```python
from build123d import *

# Parameters (mm, degrees)
SKETCH1_R                       = 32.5
EXTRUDE1_DEPTH                  = 18.9992
CHAMFER1_SIZE                   = 4.57
M3X0_5_TAPPED_HOLE3_D           = 2.5
M3X0_5_TAPPED_HOLE3_DEPTH       = 7.8486
M3X0_5_TAPPED_HOLE3_CBORE_D     = 3
M3X0_5_TAPPED_HOLE3_CBORE_DEPTH = 6.35
M3X0_5_TAPPED_HOLE3_TIP         = 0.751075774
M5X0_8_TAPPED_HOLE1_D           = 4.2
M5X0_8_TAPPED_HOLE1_DEPTH       = 27.94
M5X0_8_TAPPED_HOLE1_CBORE_D     = 5
M5X0_8_TAPPED_HOLE1_CBORE_DEPTH = 7.62
M5X0_8_TAPPED_HOLE1_TIP         = 1.2618073
HOLE1_D                         = 3.048
HOLE1_DEPTH                     = 6.35
HOLE1_CBORE_D                   = 7.874
HOLE1_CBORE_DEPTH               = 0.254
HOLE1_TIP                       = 0.915711583
SKETCH2_R                       = 31.6865
EXTRUDE2_DEPTH                  = 1.00076


with BuildPart() as part:
    # Sketch1 → Extrude1 (new body)
    with BuildSketch(Plane(origin=(0, 0, 0), x_dir=(1, 0, 0), z_dir=(0, 1, 0))):
        with Locations(Location((0, 0, 0), (0, 0, 270))):  # turned: the seam where the file's is
            Circle(SKETCH1_R)
    extrude(amount=EXTRUDE1_DEPTH)

    # Sketch3 → Cut-Revolve1 (revolve, cut)
    with BuildSketch(Plane.XY, mode=Mode.PRIVATE) as cut_revolve1_sk:
        with BuildLine():
            Line((2.3876, 13.463763428), (2.3876, 12.7508))
            Line((2.3876, 12.7508), (0, 12.7508))
            Line((0, 12.7508), (0, 18.9992))
            Line((0, 18.9992), (6.470525878, 18.9992))
            ThreePointArc((6.470525878, 18.9992), (5.220905936, 15.647420055), (2.3876, 13.463763428))
        make_face()
    revolve(cut_revolve1_sk.sketch.rotate(Axis((0, 18.9992, 0), (0, -1, 0)), 90), axis=Axis((0, 18.9992, 0), (0, -1, 0)), mode=Mode.SUBTRACT)  # turned: the seam where the file's is

    # Chamfer1
    chamfer1_edges = [part.edges().sort_by_distance(p)[0] for p in [
        (0, 18.9992, -32.5),
    ]]
    chamfer(chamfer1_edges, length=CHAMFER1_SIZE)

    # M3x0.5 Tapped Hole3
    with Locations(Plane(origin=(0, 18.9992, 0), x_dir=(-1, 0, 0), z_dir=(0, 1, 0))):
        with Locations((-5.3975, -9.348744234), (10.795, 0), (-5.3975, 9.348744234)):
            CounterBoreHole(M3X0_5_TAPPED_HOLE3_D / 2, M3X0_5_TAPPED_HOLE3_CBORE_D / 2, M3X0_5_TAPPED_HOLE3_CBORE_DEPTH, depth=M3X0_5_TAPPED_HOLE3_DEPTH)
            with Locations((0, 0, -(M3X0_5_TAPPED_HOLE3_DEPTH + M3X0_5_TAPPED_HOLE3_TIP / 2))):  # 118° drill point
                Cone(0, M3X0_5_TAPPED_HOLE3_D / 2, M3X0_5_TAPPED_HOLE3_TIP, mode=Mode.SUBTRACT)

    # M5x0.8 Tapped Hole1
    with Locations(Plane(origin=(32.5, 6.6802, 0), x_dir=(0, 0, 1), z_dir=(1, 0, 0))):
        with Locations((0, 0)):
            CounterBoreHole(M5X0_8_TAPPED_HOLE1_D / 2, M5X0_8_TAPPED_HOLE1_CBORE_D / 2, M5X0_8_TAPPED_HOLE1_CBORE_DEPTH, depth=M5X0_8_TAPPED_HOLE1_DEPTH)
            with Locations((0, 0, -(M5X0_8_TAPPED_HOLE1_DEPTH + M5X0_8_TAPPED_HOLE1_TIP / 2))):  # 118° drill point
                Cone(0, M5X0_8_TAPPED_HOLE1_D / 2, M5X0_8_TAPPED_HOLE1_TIP, mode=Mode.SUBTRACT)

    # Hole1
    with Locations(Plane(origin=(32.5, 6.6802, 0), x_dir=(0, 0, 1), z_dir=(1, 0, 0))):
        with Locations((0, 0)):
            CounterBoreHole(HOLE1_D / 2, HOLE1_CBORE_D / 2, HOLE1_CBORE_DEPTH, depth=HOLE1_DEPTH)
            with Locations((0, 0, -(HOLE1_DEPTH + HOLE1_TIP / 2))):  # 118° drill point
                Cone(0, HOLE1_D / 2, HOLE1_TIP, mode=Mode.SUBTRACT)

    # Sketch2 → Extrude2 (add)
    with BuildSketch(Plane.XZ):
        with Locations(Location((0, 0, 0), (0, 0, 90))):  # turned: the seam where the file's is
            Circle(SKETCH2_R)
    extrude(amount=EXTRUDE2_DEPTH)


solid = part.part
```
Geometry check sheet. Reference: the model listing, model coordinates, mm. A direction names the side the tool comes from. Coordinates: 2 decimals unless noted, no trailing zeros. Put each result on its own line as item: value.
1) Thickness scan on line 1 (Y direction, x = 27.25, z = 0); line 2 (Y direction, x = 32.3, z = 0); line 3 (Z direction, x = 29.5, y = 5.25). Record the ranges inside material, lowest first.
Result set:
line 1: y = -1 to 4.18, 9.18 to 19
line 2: y = 0 to 2.74, 10.62 to 14.63
line 3: z = -13.64 to -2.05, 2.05 to 13.64
2) Gauge pin test, flat ends, axial feed: pin 1 Ø4 at (x, y) = (8.5, 5.5) entering from +Z; pin 2 Ø5.5 at (y, z) = (6.5, -1) entering from +X; pin 3 Ø0.9 at (x, z) = (-10.5, 0.5) entering from +Y. Record the tip position at first contact, or that the pin passes through.
Result set:
pin 1: stops at z = 31.84
pin 2: stops at x = 32.25
pin 3: stops at y = 11.02
3) Tool access check on faces 4 (the flat face through (7, 18.999, 0)), 5 (the flat face through (0, 12.751, 0)). Record the directions out of +Z, -Z, +X, -X, +Y, -Y that give a thin tool (end or side, any length) a straight path to the whole face; none if there is none.
Result set:
face 4: +Z, -Z, +X, -X, +Y
face 5: +Y
4) Cross-section at A-A on y = 15.75. Count the separate pieces of the cut face and the enclosed holes in it, plus the area to 3 significant figures.
Result set:
separate pieces: 1
enclosed holes: 4
area: 2,940 mm^2
5) Release check for a two-part mould opening along Z. For faces 1 (the cylindrical face through (19.281, -0.493, -25.145)), 2 (the cylindrical face through (28.61, 9.12, -0.54)), 3 (the flat face through (-31.1, 0, 7.1)) record: released by +Z, released by -Z, zero draft, split by the parting line, or undercut.
Result set:
face 1: split by the parting line
face 2: undercut
face 3: zero draft
